from build123d import *

# Parameters (mm, degrees)
SKETCH2_R           = 13.49375
SKETCH2_R_2         = 11.1125
BOSS_EXTRUDE1_DEPTH = 35.71875
SKETCH5_R           = 13.335
BOSS_EXTRUDE2_DEPTH = 30.32
CUT_EXTRUDE1_REACH  = 44.069
SKETCH6_R           = 10.6807


with BuildPart() as part:
    # Sketch2 → Boss-Extrude1 (new body, symmetric)
    with BuildSketch(Plane(origin=(0, 0, 0), x_dir=(0, 0, -1), z_dir=(1, 0, 0))):
        Circle(SKETCH2_R)
        Circle(SKETCH2_R_2, mode=Mode.SUBTRACT)
    extrude(amount=BOSS_EXTRUDE1_DEPTH, both=True)

    # Sketch5 → Boss-Extrude2 (add)
    with BuildSketch(Plane(origin=(0, 28.575, 0), x_dir=(1, 0, 0), z_dir=(0, 1, 0))):
        Circle(SKETCH5_R)
    extrude(amount=-BOSS_EXTRUDE2_DEPTH)

    # Sketch6 → Cut-Extrude1 (cut, up to next)
    with BuildSketch(Plane(origin=(0, 28.575, 0), x_dir=(1, 0, 0), z_dir=(0, 1, 0)), mode=Mode.PRIVATE) as cut_extrude1_sk1:
        Circle(SKETCH6_R)
    cut_extrude1_tool1 = extrude(cut_extrude1_sk1.sketch, amount=-CUT_EXTRUDE1_REACH, mode=Mode.PRIVATE) & part.part
    add(cut_extrude1_tool1.solids().sort_by_distance((0, 28.575, 0))[0], mode=Mode.SUBTRACT)


solid = part.part
The listing builds one solid part. Answer for the finished solid, in the listing's coordinates (mm). A direction names the side the tool comes from. Give positions to 0.01 mm unless a question says otherwise; leave off trailing zeros. Write each loop counter-clockwise with the first axis right and the second up, starting at its lowest first coordinate (ties: lowest second). Pieces come first, ordered by that corner, then holes. Notation, with made-up numbers: (59, 5.25) - (82, 5.25) arc R29 cw to (82, 39.25) - close; hole circle Ø1 at (28, 48). An arc over 180 degrees is marked (long way). Use a Markdown table: item, result.
1. For a pull along Y with two mould halves and no side action, classify faces 4 (the cylindrical face through (9.866, 13.627, 4.091)), 5 (the flat face through (0, 28.575, -11)), 6 (the cylindrical face through (0.5, -13.17, 2.93)), 7 (the cylindrical face through (13.334, 3.346, 0.185)) as released by +Y, released by -Y, zero draft, split by the parting line, or undercut.
Values follow:
| item | result |
|---|---|
| face 4 | zero draft |
| face 5 | released by +Y |
| face 6 | split by the parting line |
| face 7 | undercut |
2. Section B-B on y = 0 is taken. Write down the section's boundary in (x, z) (1 decimal), plus the area to 3 significant figures.
Values follow:
| item | result |
|---|---|
| outline | (-35.7, -13.5) - (35.7, -13.5) - (35.7, -11.1) - (7.4, -11.1) arc R13.3 ccw to (7.4, 11.1) - (35.7, 11.1) - (35.7, 13.5) - (-35.7, 13.5) - (-35.7, 11.1) - (-7.4, 11.1) arc R13.3 ccw to (-7.4, -11.1) - (-35.7, -11.1) - close; hole circle Ø21.4 at (0, 0) |
| area | 496 mm² |
3. Each of these flat-tipped pins is pushed along its axis until it touches: P1, Ø5, axis at x = 23, y = -9, coming from the -Z side (3 decimals); P2, Ø12, axis at x = -7, z = 8, coming from the -Y side; P3, Ø1.5, axis at y = 19, z = 5.5, coming from the +X side. Where does it stop, or does it pass through?
Values follow:
| item | result |
|---|---|
| P1 | stops at z = -11.825 |
| P2 | stops at y = -13.34 |
| P3 | stops at x = 12.46 |
4. Section D-D on y = -7 is taken. Write down the section's boundary in (x, z), plus the area to 3 significant figures.
Values follow:
| item | result |
|---|---|
| outline | (-35.72, -11.54) - (35.72, -11.54) - (35.72, -8.63) - (-35.72, -8.63) - close; (-35.72, 8.63) - (35.72, 8.63) - (35.72, 11.54) - (-35.72, 11.54) - close |
| area | 415 mm² |
5. Section A-A on z = 0 is taken. Write down the section's boundary in (x, y) (1 decimal).
Values follow:
| item | result |
|---|---|
| outline | (-35.7, -13.5) - (35.7, -13.5) - (35.7, -11.1) - (-35.7, -11.1) - close; (-35.7, 11.1) - (-13.3, 11.1) - (-13.3, -1.7) - (-10.7, -1.7) - (-10.7, 28.6) - (-13.3, 28.6) - (-13.3, 13.5) - (-35.7, 13.5) - close; (10.7, -1.7) - (13.3, -1.7) - (13.3, 11.1) - (35.7, 11.1) - (35.7, 13.5) - (13.3, 13.5) - (13.3, 28.6) - (10.7, 28.6) - close |
6. A tool of negligible diameter and unlimited length cuts with its end or side. For faces 1 (the cylindrical face through (6.15, 18.44, 11.83)), 2 (the cylindrical face through (-0.5, -10.85, 2.41)), 3 (the flat face through (35.719, 10.1, 5.1)), from which of +Z, -Z, +X, -X, +Y, -Y can it reach the whole face along a straight path? Write none if from no direction.
Values follow:
| item | result |
|---|---|
| face 1 | +Y |
| face 2 | none |
| face 3 | +Z, -Z, +X, +Y, -Y |
7. Find the intervals of material crossed by probe 1 along Z at (x, y) = (0, 12) (3 decimals); probe 2 along Y at (x, z) = (17, 0.5), in increasing order. Write a range as from..to.
Values follow:
| item | result |
|---|---|
| probe 1 | z = -13.335..-10.681, 10.681..13.335 |
| probe 2 | y = -13.48..-11.1, 11.1..13.48 |
